Geometry: final body of the model. Coordinates: model frame, mm. A direction names the side the tool comes from. Coordinates: 2 decimals unless noted, no trailing zeros. Order: outer loops, then holes, each group sorted by start corner. A loop starts at its lowest first (then second) coordinate and runs counter-clockwise, first axis right, second up. Notation, with made-up numbers: (62, 71.25) - (70, 71.25) arc R9 ccw to (70, 84.25) - close; hole circle Ø3 at (45, 7). An arc over 180 degrees is marked (long way). Use a Markdown table: item, result. Add a question column.
```python
from build123d import *

# Parameters (mm, degrees)
F0_W     = 8.1289224327
F0_H     = 36.6465272382
F1_DEPTH = 25.4


with BuildPart() as f1:
    # F0 (on Front) → F1 (new body)
    with BuildSketch(Plane.XZ):
        Polygon((-24.8146168888, 40.9678071737), (-66.3149282336, 40.9678071737), (-66.3149282336, 14.6492579952), (-58.186005801, 14.6492579952), (-58.186005801, -21.997269243), (-66.3149282336, -21.997269243), (-66.3149282336, -38.6094748974), (-24.8146168888, -38.6094748974), align=None)
        with Locations((-62.2504670173, -3.6740056239)):
            Rectangle(F0_W, F0_H)
        Polygon((-66.3149282336, -21.997269243), (-66.3149282336, 14.6492579952), (-214.7748172283, 14.6492579952), (-214.5942430103, 14.1340185696), (-209.6407413483, 6.0107740574), (-195.9499269724, 6.0107740574), (-195.9499269724, 0), (-171.5631484985, -21.997269243), align=None)
        Polygon((-214.5942430103, 14.1340185696), (-214.7748172283, 14.6492579952), (-214.7748172283, 14.4301421254), align=None)
        Polygon((-214.7748172283, -21.997269243), (-171.5631484985, -21.997269243), (-195.9499269724, 0), (-209.6407413483, 0), (-214.5942430103, 14.1340185696), (-214.7748172283, 14.4301421254), align=None)
    extrude(amount=F1_DEPTH)


solid = f1.part
```
1) Line query: line 1 (Z direction, x = -138, y = -8); line 2 (X direction, y = -20, z = 13); line 3 (X direction, y = -13.25, z = 17). Output: solid intervals per line, ascending. Write a range as from..to.
2) Draft query along X for faces 1 (the flat face through (-203, -13, 6.011)), 2 (the flat face through (-100, 0, 2)), 3 (the flat face through (-24.815, -13, 1)), 4 (the flat face through (-214.775, -13, -3)). Return one class per face: released by +X, released by -X, zero draft, split by the parting line, or undercut.
3) Section query A-A (x = -202.5). Return the cut outline in (y, z).
4) Access query for faces 5 (the flat face through (-142, -13, -21.997)), 6 (the flat face through (-100, -25.4, 2)), 7 (the flat face through (-45, -13, 40.968)), 8 (the flat face through (-140, -13, 14.649)), 9 (the flat face through (-195.95, -13, 3)). Directions: +Z, -Z, +X, -X, +Y, -Y. A direction counts if a zero-diameter tool reaches every point of the face in a straight line with its end or side. Return the directions, or none.
5) First-contact query: pin 1 (11 mm diameter, centred on x = -205, y = -16, fed in from -Z); pin 2 (11 mm diameter, centred on x = -204, y = -10, fed in from +Z); pin 3 (7.5 mm diameter, centred on y = -10, z = 29, fed in from -X); pin 4 (4 mm diameter, centred on x = -56.5, z = 7, fed in from +Y). Flat tips, straight axial feed; report the tip coordinate or a pass-through.
6) Section query D-D (z = 27). Return the cut outline in (x, y).
7) Section query B-B (y = -7.5). Return the cut outline in (x, z).
8) Section query C-C (x = -126). Return the cut outline in (y, z), and give its area (3 significant figures).
From the geometry:
| question | item | result |
|---|---|---|
| 1 | line 1 | z = -22..14.65 |
| 1 | line 2 | x = -214.77..-214.2, -213.9..-24.81 |
| 1 | line 3 | x = -66.31..-24.81 |
| 2 | face 1 | undercut |
| 2 | face 2 | zero draft |
| 2 | face 3 | released by +X |
| 2 | face 4 | released by -X |
| 3 | outline | (-25.4, -22) - (0, -22) - (0, 0) - (-25.4, 0) - close; (-25.4, 6.01) - (0, 6.01) - (0, 14.65) - (-25.4, 14.65) - close |
| 4 | face 5 | -Z, -X, +Y, -Y |
| 4 | face 6 | +Z, -Z, +X, -X, -Y |
| 4 | face 7 | +Z, +X, -X, +Y, -Y |
| 4 | face 8 | +Z, -X, +Y, -Y |
| 4 | face 9 | +Y, -Y |
| 5 | pin 1 | stops at z = -22 |
| 5 | pin 2 | stops at z = 14.65 |
| 5 | pin 3 | stops at x = -66.31 |
| 5 | pin 4 | stops at y = 0 |
| 6 | outline | (-66.31, -25.4) - (-24.81, -25.4) - (-24.81, 0) - (-66.31, 0) - close |
| 7 | outline | (-214.77, -22) - (-66.31, -22) - (-66.31, -38.61) - (-24.81, -38.61) - (-24.81, 40.97) - (-66.31, 40.97) - (-66.31, 14.65) - (-214.77, 14.65) - close; hole (-214.59, 14.13) - (-209.64, 0) - (-195.95, 0) - (-195.95, 6.01) - (-209.64, 6.01) - close |
| 8 | outline | (-25.4, -22) - (0, -22) - (0, 14.65) - (-25.4, 14.65) - close |
| 8 | area | 931 mm^2 |
